Can you work these out from the model? Positions are in its coordinate system, mm. A direction names the side the tool comes from. Round coordinates to 2 decimals unless told otherwise and drop trailing zeros. Loops run counter-clockwise (first coordinate to the right, second up) from the corner with the lowest first, then second, coordinate; pieces in that order, holes last. Notation, with made-up numbers: (-17, -17.5) -> (8, -17.5) arc R8 cw to (8, -9.5) -> close; hole circle Ø3 at (84.25, 12.5). An arc over 180 degrees is marked (long way). Write item = value, one per line.
Autodesk Inventor part; units mm, degrees
ref_plane "YZ Plane" through (0, 0, 0) normal (1, 0, 0) x (0, 1, 0)
ref_plane "XZ Plane" through (0, 0, 0) normal (0, 1, 0) x (-1, 0, 0)
ref_plane "XY Plane" through (0, 0, 0) normal (0, 0, 1) x (1, 0, 0)
sketch "Sketch1" plane through (0, 0, 0) normal (0, 1, 0) x (-1, 0, 0)
  line L0 (21.324, 10.54) -> (-21.324, 10.54)
  line L1 (-21.324, -33.91) -> (-15.724, -33.91)
  circle A0 centre (-23.749, -25.782) radius 1.524
  circle A1 centre (-23.749, 7.365) radius 1.524
  circle A2 centre (23.749, 7.365) radius 1.524
  circle A3 centre (10.414, -37.085) radius 1.524
  circle A4 centre (-10.414, -37.085) radius 1.524
  line L2 (-29.924, 14.3694) -> (-29.924, -45.6306)
  line L3 (29.924, 14.3694) -> (29.924, -45.6306)
  line L4 (-29.924, 14.3694) -> (29.924, 14.3694)
  line L5 (-21.324, -33.91) -> (-7.574, -33.91)
  line L6 (-7.574, -33.91) -> (-7.574, -40.26)
  line L7 (-7.574, -40.26) -> (7.574, -40.26)
  line L8 (29.924, -45.6306) -> (-29.924, -45.6306)
  line L9 (-21.324, 10.54) -> (21.324, 10.54)
  circle A5 centre (-23.749, 7.365) radius 1.524
  circle A6 centre (23.749, 7.365) radius 1.524
  circle A7 centre (-23.749, -25.782) radius 1.524
  circle A8 centre (10.414, -37.085) radius 1.524
  circle A9 centre (-10.414, -37.085) radius 1.524
  line L10 (-21.324, -8.1306) -> (21.324, -8.1306)
  line L11 (-21.324, -12.8806) -> (21.324, -12.8806)
  line L12 (-21.324, 10.54) -> (-21.324, -8.1306)
  line L13 (-21.324, -12.8806) -> (-21.324, -33.91)
  line L14 (21.324, -33.91) -> (21.324, -12.8806)
  line L15 (21.324, -8.1306) -> (21.324, 10.54)
  line L16 (21.324, -33.91) -> (7.574, -33.91)
  line L17 (7.574, -33.91) -> (7.574, -40.26)
  point P0 (0, 0)
  point P1 (-14.449, -33.91)
  dimension "d6" = 60
  dimension "d9" = 13.75
  dimension "d11" = 56.1706
  dimension "d12" = 37.5
  dimension "d13" = 32.75
  dimension "d14" = 51.248
  dimension "d15" = 8.6
extrude "Extrusion1" add sketch "Sketch1" along normal blind 7.62
sketch "Sketch2" plane through (0, 0, 0) normal (0, -1, 0) x (1, 0, 0)
  line L0 (21.324, 10.54) -> (-21.324, 10.54)
  line L1 (0, 10.54) -> (-26.924, 10.54)
  line L2 (-26.924, 10.54) -> (-26.924, -40.26)
  line L3 (-26.924, -40.26) -> (26.924, -40.26)
  line L4 (26.924, -40.26) -> (26.924, 10.54)
  line L5 (26.924, 10.54) -> (0, 10.54)
  point P0 (0, 0)
  dimension "d18" = 26.924
  dimension "d19" = 50.8
  dimension "d20" = 53.848
extrude "Extrusion2" cut sketch "Sketch2" against normal blind 1.5875
fillet "Fillet1" radius 5.08 4 edges at (29.924, 3.81, 14.3694) (-29.924, 3.81, 14.3694) (29.924, 3.81, -45.6306) (-29.924, 3.81, -45.6306)
sketch "Sketch3" plane through (0, 0, 0) normal (0, -1, 0) x (1, 0, 0)
  line L0 (-24.844, 14.3694) -> (24.844, 14.3694)
  line L1 (-9.9342, 14.3694) -> (-9.9342, 10.54)
  line L2 (-29.924, -40.5506) -> (-29.924, 9.2894)
  line L3 (22.177, 14.3694) -> (22.177, 10.54)
  line L4 (-26.924, 10.54) -> (26.924, 10.54)
  line L5 (29.924, 9.2894) -> (29.924, -40.5506)
  line L6 (-9.9342, 14.3694) -> (22.177, 14.3694)
  line L7 (22.177, 10.54) -> (-9.9342, 10.54)
  point P0 (0, 0)
  dimension "d24" = 19.9898
  dimension "d25" = 7.747
extrude "Extrusion3" add sketch "Sketch3" along normal blind 4.2926
sketch "Sketch4" plane through (0, 1.5875, 0) normal (0, -1, 0) x (1, 0, 0)
  line L0 (21.324, -33.91) -> (21.324, -12.8806)
  line L1 (26.924, -40.26) -> (-26.924, -40.26)
  line L2 (-21.324, -33.91) -> (-7.574, -33.91)
  line L3 (-26.924, -40.26) -> (-14.224, -40.26)
  line L4 (-15.7226, -33.91) -> (-26.924, -33.91)
  line L5 (-26.924, -33.91) -> (-26.924, -40.26)
  line L6 (7.574, -33.91) -> (21.324, -33.91)
  line L7 (26.924, -40.26) -> (14.224, -40.26)
  line L8 (15.7226, -33.91) -> (26.924, -33.91)
  line L9 (26.924, -33.91) -> (26.924, -40.26)
  line L10 (-14.224, -40.26) -> (-14.224, -35.4086)
  circle A0 centre (-10.414, -37.085) radius 1.524
  line L11 (-15.7226, -33.91) -> (-14.224, -35.4086)
  line L12 (14.224, -40.26) -> (14.224, -35.4086)
  circle A1 centre (10.414, -37.085) radius 1.524
  line L13 (14.224, -35.4086) -> (15.7226, -33.91)
  point P0 (0, 0)
  dimension "d42" = 11.2014
  dimension "d43" = 11.2014
  dimension "d44" = 4.8514
  dimension "d45" = 3.81
  dimension "d46" = 4.8514
  dimension "d48" = 3.81
  dimension "d49" = 6.35
  dimension "d50" = 6.35
extrude "Extrusion4" add sketch "Sketch4" along normal blind 1.5875 contours L1 L5 L4 L2 L11 L10 | L1 L12 L13 L6 L8 L9
sketch "Sketch5" plane through (0, 0, 0) normal (0, -1, 0) x (1, 0, 0)
  line L0 (-14.224, -40.26) -> (-14.224, -35.4086)
  line L1 (-15.7226, -33.91) -> (-26.924, -33.91)
  line L2 (-26.924, -33.91) -> (-26.924, 10.54)
  line L3 (0, -57.6306) -> (0, 26.3694)
  line L4 (-26.924, 10.54) -> (-9.9342, 10.54)
  line L5 (-24.844, 14.3694) -> (-9.9342, 14.3694)
  line L6 (-29.924, -40.5506) -> (-29.924, 9.2894)
  circle A0 centre (-21.3233, -39.7647) radius 1.5875
  circle A1 centre (21.3233, -39.7647) radius 1.5875
  point P0 (0, 0)
  dimension "d101" = 3.175
  dimension "d102" = 5.8547
  dimension "d104" = 7.0993
extrude "Extrusion6" cut sketch "Sketch5" against normal up to next
properties part number "front-cam"
1. Suppose I cut it at C-C, the plane y = 4.5. Count the separate pieces of the cut face and the enclosed holes in it, and give its area (3 significant figures).
Entries:
separate_pieces = 1
enclosed_holes = 9
area = 1,730 mm²
2. I'm going to push flat-ended pins straight in: pin 1 (4 mm diameter, centred on x = -22.5, z = -31, fed in from -Y); pin 2 (2 mm diameter, centred on x = -4.5, y = -1.5, fed in from -Z); pin 3 (1.9 mm diameter, centred on y = -3, z = 13, fed in from +X). Where does each tip first touch, or does it pass through?
Entries:
pin_1 = 1.59
pin_2 = 10.54
pin_3 = 22.18
3. We'd pull the mould along Z, two halves only. Please class faces 1 (the flat face through (0, 2, 10.54)), 2 (the flat face through (29.924, 4, -15)), 3 (the flat face through (0, 4, -45.631)): released by +Z, released by -Z, zero draft, split by the parting line, or undercut.
Entries:
face_1 = undercut
face_2 = zero draft
face_3 = released by -Z
4. Suppose I cut it at A-A, the plane z = -14. List the corners of the cut face in (x, y) for me.
Entries:
outline = (-29.92, 0) -> (-26.92, 0) -> (-26.92, 1.59) -> (-21.32, 1.59) -> (-21.32, 7.62) -> (-29.92, 7.62) -> close; (21.32, 1.59) -> (26.92, 1.59) -> (26.92, 0) -> (29.92, 0) -> (29.92, 7.62) -> (21.32, 7.62) -> close
5. Suppose I cut it at B-B, the plane x = -17.5. List the corners of the cut face in (y, z) for me, and give its area (3 significant figures).
Entries:
outline = (0, -45.63) -> (7.62, -45.63) -> (7.62, -33.91) -> (0, -33.91) -> close; (0, 10.54) -> (7.62, 10.54) -> (7.62, 14.37) -> (0, 14.37) -> close; (1.59, -12.88) -> (7.62, -12.88) -> (7.62, -8.13) -> (1.59, -8.13) -> close
area = 147 mm²
6. For faces 4 (the flat face through (21.324, 5, -23)), 5 (the flat face through (22.177, -2, 12)), 6 (the flat face through (-9.934, -2, 12)), 7 (the flat face through (-14.98, 0.8, -34.65)), which set-ups out of +Z, -Z, +X, -X, +Y, -Y let a thin tool reach every point of the face, with its end or its side?
Entries:
face_4 = +Y, -Y
face_5 = +Z, -Z, +X, -Y
face_6 = +Z, -Z, -X, -Y
face_7 = -Y
7. Suppose I cut it at D-D, the plane x = -1. List the corners of the cut face in (y, z) for me, and give its area (3 significant figures).
Entries:
outline = (-4.29, 10.54) -> (7.62, 10.54) -> (7.62, 14.37) -> (-4.29, 14.37) -> close; (0, -45.63) -> (7.62, -45.63) -> (7.62, -40.26) -> (0, -40.26) -> close; (1.59, -12.88) -> (7.62, -12.88) -> (7.62, -8.13) -> (1.59, -8.13) -> close
area = 115 mm²
8. I need wall thicknesses on line 1 (Z direction, x = 7.5, y = 5); line 2 (Z direction, x = 13, y = 5.5); line 3 (X direction, y = 4.25, z = 5.5). Which ranges of each line are inside material? Lowest first, please. Write a range as [from, to].
Entries:
line_1 = [-45.63, -40.26], [-12.88, -8.13], [10.54, 14.37]
line_2 = [-45.63, -33.91], [-12.88, -8.13], [10.54, 14.37]
line_3 = [-29.92, -21.32], [21.32, 29.92]
